Check sheet for the modelled part. Datum: model origin and axes. Units: mm. A direction names the side the tool comes from. Round coordinates to 2 decimals unless told otherwise and drop trailing zeros. Loops run counter-clockwise (first coordinate to the right, second up) from the corner with the lowest first, then second, coordinate; pieces in that order, holes last. Notation, with made-up numbers: (28.5, -24) -> (76.5, -24) arc R25 ccw to (76.5, 7) -> close; hole circle Ø1 at (46.5, 8.5). An arc over 180 degrees is marked (long way). One line per item, written item: value. Start each with the question number.
1. Go/stop test with flat-tipped pins: pin 1 (12 mm diameter, centred on y = 23.56, z = -15, fed in from -X); pin 2 (2.5 mm diameter, centred on x = 8, z = -5.5, fed in from -Y); pin 3 (9 mm diameter, centred on x = 14, z = 22, fed in from -Y). Record where each tip stops, or that it passes through.
2. Set-up check for faces 1 (the face through (-19, 100, -14)), 2 (the face through (25, -7, -21.975)), 3 (the face through (10, 16, -25.05)): record each of +Z, -Z, +X, -X, +Y, -Y from which the full face is reachable in a straight line by a thin tool's end or side.
3. Cross-section at D-D on x = 16.5. Record the cut outline in (y, z), then the cut area to 3 significant figures.
4. Release check for a two-part mould opening along Y. For faces 4 (the face through (23, 112, -14)), 5 (the face through (15, 85, -45)), 6 (the face through (-19.23, 106.06, -14.37)), 7 (the face through (10, 15, -4.95)) record: +Y half, -Y half, draft (parallel to the pull), parting line (faces both ways), or undercut.
5. Cross-section at A-A on y = 15.06. Record the cut outline in (x, z) (3 decimals), then the cut area to 4 significant figures.
6. Material ranges on L1, parallel to Z at x = 25, y = 15; L2, parallel to Y at x = 25, z = -15 (3 decimals); L3, parallel to Y at x = 26.75, z = -15 (3 decimals), recorded low to high.
7. Cross-section at C-C on z = -37. Record the cut outline in (x, y), then the cut area to 3 significant figures.
8. Cross-section at B-B on z = -15. Count the separate pieces of the cut face and the enclosed holes in it, then the cut area to 3 significant figures.
Autodesk Inventor part; units mm, degrees
ref_plane "Work Plane1" through (0, 0, -15) normal (0, 0, 1) x (1, 0, 0)
ref_plane "YZ Plane" through (0, 0, 0) normal (1, 0, 0) x (0, 1, 0)
ref_plane "XZ Plane" through (0, 0, 0) normal (0, 1, 0) x (-1, 0, 0)
sketch "Sketch1" plane through (0, 0, 0) normal (0, 0, 1) x (1, 0, 0)
  line L0 (0, 0) -> (25, 0)
  line L1 (25, 0) -> (25, 40)
  line L2 (25, 40) -> (0, 40)
  line L3 (0, 40) -> (0, 0)
  dimension "d1" = 25
  dimension "d2" = 40
  dimension "d3" = 25
extrude "Extrusion1" add sketch "Sketch1" against normal blind 30
sketch "Sketch2" plane through (25, 0, 0) normal (1, 0, 0) x (0, 0, -1)
  line L0 (0, 0) -> (30, 0)
  circle A0 centre (15, 6.56) radius 2.46
extrude "Extrusion2" cut sketch "Sketch2" against normal blind 30
sketch "Sketch3" plane through (0, 0, 0) normal (-1, 0, 0) x (0, 0, 1)
  line L0 (0, 0) -> (-30, 0)
  line L1 (-25.05, 0) -> (-4.95, 0)
  line L2 (-4.95, 0) -> (-4.95, 33.12)
  line L3 (-4.95, 33.12) -> (-25.05, 33.12)
  line L4 (-25.05, 33.12) -> (-25.05, 0)
  dimension "d11" = 20.1
extrude "Extrusion3" cut sketch "Sketch3" against normal blind 20
sketch "Sketch4" plane through (0, 0, 0) normal (0, -1, 0) x (1, 0, 0)
  line L0 (20, -4.95) -> (20, -25.05)
  line L1 (20, -15) -> (25, -15)
  line L2 (25, 0) -> (25, -30)
  line L3 (20, -8.025) -> (25, -8.025)
  line L4 (25, -8.025) -> (25, -21.975)
  line L5 (25, -21.975) -> (20, -21.975)
  line L6 (20, -21.975) -> (20, -8.025)
  line L7 (20, -8.025) -> (25, -21.975) construction
  line L8 (25, -8.025) -> (20, -21.975) construction
  line L9 (25, -12.54) -> (25, -17.46)
  point P0 (0, 0)
  point P1 (22.5, -15)
  dimension "d14" = 13.95
extrude "Extrusion4" add sketch "Sketch4" along normal blind 15
sketch "Sketch5" plane through (20, 0, 0) normal (-1, 0, 0) x (0, 0, 1)
  circle A0 centre (-15, 6.56) radius 2.46
  circle A1 centre (-15, 6.56) radius 4.7025
  circle A2 centre (-15, 6.56) radius 2.46
  circle A3 centre (-15, 6.56) radius 2.46
  point P0 (0, 0)
  dimension "d17" = 9.405
extrude "Extrusion5" cut sketch "Sketch5" against normal blind 2.1
sketch "Sketch6" plane through (25, 0, 0) normal (1, 0, 0) x (0, 0, -1)
  circle A0 centre (15, 6.56) radius 4.7025
  line L0 (15, 6.56) -> (15, 23.56)
  circle A1 centre (15, 23.56) radius 2.46
  point P0 (0, 0)
  dimension "d20" = 17
  dimension "d21" = 4.92
extrude "Extrusion6" cut sketch "Sketch6" against normal blind 10 contours A1
sketch "Sketch7" plane through (20, 0, 0) normal (-1, 0, 0) x (0, 0, 1)
  circle A0 centre (-15, 23.56) radius 2.46
  circle A1 centre (-15, 23.56) radius 4.7025
  point P0 (0, 0)
  dimension "d24" = 9.405
extrude "Extrusion7" cut sketch "Sketch7" against normal blind 2.1
sketch "Sketch9" plane through (25, 0, 0) normal (1, 0, 0) x (0, 0, -1)
  circle A0 centre (15, 6.56) radius 2.46
  circle A1 centre (15, 6.56) radius 2.46
  circle A2 centre (15, 23.56) radius 2.46
  circle A3 centre (15, 23.56) radius 2.46
  line L0 (30, 40) -> (30, 0)
  line L1 (30, 0) -> (30, 40)
  line L2 (30, 40) -> (0, 40)
  line L3 (0, 40) -> (0, 0)
  line L4 (0, 0) -> (8.025, 0)
  line L5 (21.975, 0) -> (21.975, -15)
  line L6 (21.975, -15) -> (8.025, -15)
  line L7 (8.025, -15) -> (8.025, 0)
  line L8 (0, 0) -> (8.025, 0)
  line L9 (21.975, 0) -> (30, 0)
extrude "Extrusion8" add sketch "Sketch9" along normal blind 5
sketch "Sketch10" plane through (0, 40, 0) normal (0, 1, 0) x (1, 0, 0)
  line L0 (0, 30) -> (30, 30)
  line L1 (30, 0) -> (0, 0)
  line L2 (0, 30) -> (30, 30)
  line L3 (30, 30) -> (30, 0)
  line L4 (30, 0) -> (0, 0)
  line L5 (0, 0) -> (0, 30)
extrude "Extrusion9" add sketch "Sketch10" along normal blind 30
sketch "Sketch12" plane through (30, 0, 0) normal (1, 0, 0) x (0, 0, -1)
  circle A0 centre (15, 6.56) radius 2.46
  line L0 (15, 6.56) -> (15, 15.06)
  circle A1 centre (15, 15.06) radius 2.525
  point P0 (0, 0)
  dimension "d31" = 8.5
  dimension "d33" = 5.05
extrude "Extrusion10" cut sketch "Sketch12" against normal blind 30 contours A1
sketch "Sketch14" plane through (0, 0, 0) normal (0, 0, 1) x (1, 0, 0)
  line L0 (30, 70) -> (0, 70)
  line L1 (0, 70) -> (0, 85)
  line L2 (-15, 100) -> (-23, 100)
  line L3 (30, 0) -> (30, 70)
  line L4 (30, 100) -> (30, 70)
  arc A0 (0, 85) -> (-15, 100) centre (-15, 85) ccw
  line L5 (-23, 120) -> (15, 120)
  line L6 (-20.5, 118) -> (-18, 110)
  line L7 (-20.5, 118) -> (-23, 120)
  line L8 (-20.5, 102) -> (-18, 110)
  line L9 (-20.5, 102) -> (-23, 100)
  line L10 (30, 105) -> (15, 120)
  line L11 (30, 105) -> (30, 100)
  point P0 (0, 0)
  point P1 (0, 100)
  dimension "d47" = 30
  dimension "d54" = 15
  dimension "d60" = 20
extrude "Extrusion12" add sketch "Sketch14" against normal blind 30
sketch "Sketch15" plane through (0, 0, -25.05) normal (-1, 0, 0) x (0, 0, 1)
  line L0 (0, 33.12) -> (20.1, 33.12)
  line L1 (20.1, 33.12) -> (20.1, 0)
  line L2 (0, 33.12) -> (20.1, 33.12)
  line L3 (20.1, 33.12) -> (20.1, 31.1)
  line L4 (20.1, 31.1) -> (0, 31.1)
  line L5 (0, 31.1) -> (0, 33.12)
  point P0 (25.05, 0)
  dimension "d57" = 2.02
extrude "Extrusion13" add sketch "Sketch15" against normal blind 20
sketch "Sketch19" plane through (0, 0, 0) normal (0, 0, 1) x (1, 0, 0)
  arc A0 (0, 85) -> (-15, 100) centre (-15, 85) ccw
  arc A1 (0, 85) -> (-15, 100) centre (-15, 85) ccw
  line L0 (-15, 100) -> (-23, 100)
  line L1 (-15, 100) -> (-23, 100)
  line L2 (-23, 100) -> (-20.5, 102)
  line L3 (-23, 100) -> (-20.5, 102)
  line L4 (-20.5, 102) -> (-18, 110)
  line L5 (-20.5, 102) -> (-18, 110)
  line L6 (-18, 110) -> (-20.5, 118)
  line L7 (-18, 110) -> (-20.5, 118)
  line L8 (-23, 120) -> (15, 120)
  line L9 (-20.5, 118) -> (-23, 120)
  line L10 (-23, 120) -> (15, 120)
  line L11 (15, 120) -> (30, 105)
  line L12 (15, 120) -> (30, 105)
  line L13 (30, 105) -> (30, 85)
  line L14 (30, 0) -> (30, 105)
  line L15 (0, 85) -> (30, 85)
  point P0 (0, 0)
extrude "Extrusion14" add sketch "Sketch19" along normal blind 30
ref_plane "Work Plane1" through (0, 0, -15) normal (0, 0, 1) x (1, 0, 0)
mirror "Mirror1" about plane through (0, 0, -15) normal (0, 0, 1) of "Extrusion14"
properties part number "16mm_x_90mm"
Taken from the geometry:
1. pin 1: stops at x = 20
1. pin 2: stops at y = 0
1. pin 3: stops at y = 85
2. face 1: +Z, -Z, -X, -Y
2. face 2: -Z, +X, -X, -Y
2. face 3: -X, -Y
3. outline: (0, -30) -> (85, -30) -> (85, -60) -> (118.5, -60) -> (118.5, 30) -> (85, 30) -> (85, 0) -> (0, 0) -> (0, -4.95) -> (31.1, -4.95) -> (31.1, -25.05) -> (0, -25.05) -> close
3. area: 4,940 mm2
4. face 4: +Y half
4. face 5: -Y half
4. face 6: undercut
4. face 7: draft
5. outline: (0, -30) -> (30, -30) -> (30, -17.525) -> (20, -17.525) -> (20, -25.05) -> (0, -25.05) -> close; (0, -4.95) -> (20, -4.95) -> (20, -12.475) -> (30, -12.475) -> (30, 0) -> (0, 0) -> close
5. area: 447.5 mm2
6. L1: z = -30 to -17.52, -12.48 to 0
6. L2: y = -15 to 4.1, 9.02 to 12.535, 17.585 to 21.1, 26.02 to 110
6. L3: y = -15 to 4.1, 9.02 to 12.535, 17.585 to 21.1, 26.02 to 108.25
7. outline: (-23, 100) -> (-15, 100) arc R15 cw to (0, 85) -> (30, 85) -> (30, 105) -> (15, 120) -> (-23, 120) -> (-20.5, 118) -> (-18, 110) -> (-20.5, 102) -> close
7. area: 1,380 mm2
8. separate pieces: 4
8. enclosed holes: 0
8. area: 3,290 mm2
